Here's how the part is built. I have some questions about the finished solid (model axes, mm). Face numbers are marked on the shaded views. A direction names the side the tool comes from. Round coordinates to 2 decimals unless told otherwise and drop trailing zeros. Write each loop counter-clockwise with the first axis right and the second up, starting at its lowest first coordinate (ties: lowest second). Pieces come first, ordered by that corner, then holes. Notation, with made-up numbers: (6, -20.5) -> (31, -20.5) arc R10 cw to (31, -7.5) -> close; hole circle Ø10 at (-8.5, 73). An arc over 180 degrees is marked (long way). Answer in a Markdown table with one row per item.
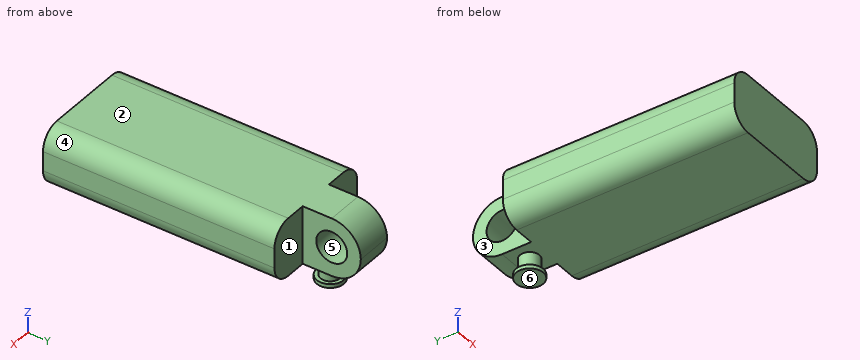
from build123d import *

# Parameters (mm, degrees)
BOSS_EXTRUDE1_DEPTH     = 29.87
SKETCH2_W               = 4.75
SKETCH2_H               = 7.5
BOSS_EXTRUDE2_DEPTH     = 7.5
CUT_EXTRUDE1_DEPTH      = 39.834199168
CUT_EXTRUDE1_DEPTH_BACK = 39.834199168
SKETCH3_R               = 2
SKETCH4_R               = 1.25
BOSS_EXTRUDE3_DEPTH     = 2
SKETCH5_R               = 1.75
BOSS_EXTRUDE4_DEPTH     = 0.5


with BuildPart() as part:
    # Sketch1 → Boss-Extrude1 (new body)
    with BuildSketch(Plane(origin=(0, 0, 0), x_dir=(1, 0, 0), z_dir=(0, 1, 0))):
        with BuildLine():
            Line((-5, 3.75), (5, 3.75))
            ThreePointArc((5, 3.75), (6.767766953, 3.017766953), (7.5, 1.25))
            Line((7.5, 1.25), (7.5, -1.25))
            ThreePointArc((7.5, -1.25), (6.767766953, -3.017766953), (5, -3.75))
            Line((5, -3.75), (-5, -3.75))
            ThreePointArc((-5, -3.75), (-6.767766953, -3.017766953), (-7.5, -1.25))
            Line((-7.5, -1.25), (-7.5, 1.25))
            ThreePointArc((-7.5, 1.25), (-6.767766953, 3.017766953), (-5, 3.75))
        make_face()
    extrude(amount=BOSS_EXTRUDE1_DEPTH)

    # Sketch2 → Boss-Extrude2 (add)
    with BuildSketch(Plane(origin=(0, 29.87, 0), x_dir=(1, 0, 0), z_dir=(0, 1, 0))):
        Rectangle(SKETCH2_W, SKETCH2_H)
    extrude(amount=BOSS_EXTRUDE2_DEPTH)

    # Sketch3 → Cut-Extrude1 (cut, two sides: drawn at the far end of the back side and taken through both)
    with BuildSketch(Plane.ZY.offset(2.375).offset(-CUT_EXTRUDE1_DEPTH_BACK)):
        with BuildLine():
            Line((-3.75, 37.37), (-3.75, 33.62))
            ThreePointArc((-3.75, 33.62), (-2.651650429, 36.271650429), (0, 37.37))
            Line((0, 37.37), (-3.75, 37.37))
        make_face()
        with BuildLine():
            ThreePointArc((0, 37.37), (2.651650429, 36.271650429), (3.75, 33.62))
            Line((3.75, 33.62), (3.75, 37.37))
            Line((3.75, 37.37), (0, 37.37))
        make_face()
        with Locations((0, 33.62)):
            Circle(SKETCH3_R)
    extrude(amount=CUT_EXTRUDE1_DEPTH + CUT_EXTRUDE1_DEPTH_BACK, mode=Mode.SUBTRACT)

    # Sketch4 → Boss-Extrude3 (add)
    with BuildSketch(Plane(origin=(0, 0, -3.75), x_dir=(-1, 0, 0), z_dir=(0, 0, -1))):
        with Locations(Location((0, 31.745, 0), (0, 0, 180))):
            Circle(SKETCH4_R)
    extrude(amount=BOSS_EXTRUDE3_DEPTH)

    # Sketch5 → Boss-Extrude4 (add)
    with BuildSketch(Plane(origin=(0, 0, -5.75), x_dir=(-1, 0, 0), z_dir=(0, 0, -1))):
        with Locations((0, 31.745)):
            Circle(SKETCH5_R)
    extrude(amount=BOSS_EXTRUDE4_DEPTH)


solid = part.part
1) We'd pull the mould along Z, two halves only. Please class the marked faces 4, 5 and 6: +Z half, -Z half, draft (parallel to the pull), parting line (faces both ways), or undercut.
Response:
| item | result |
|---|---|
| face 4 | +Z half |
| face 5 | undercut |
| face 6 | -Z half |
2) I want a section at A-A, the plane x = 0. List the corners of the cut face in (y, z) for me (3 decimals), and give its area (3 significant figures).
Response:
| item | result |
|---|---|
| outline | (0, -3.75) -> (30.495, -3.75) -> (30.495, -5.75) -> (29.995, -5.75) -> (29.995, -6.25) -> (33.495, -6.25) -> (33.495, -5.75) -> (32.995, -5.75) -> (32.995, -3.75) -> (33.62, -3.75) arc R3.75 ccw to (33.62, 3.75) -> (0, 3.75) -> close; hole circle Ø4 at (33.62, 0) |
| area | 268 mm^2 |
3) For pin 1 (2.5 mm diameter, centred on x = 5.5, z = 0.5, fed in from +Y); pin 2 (2 mm diameter, centred on y = 34.5, z = 1, fed in from -X) (3 decimals); pin 3 (5 mm diameter, centred on x = -2, y = 20, fed in from -Z), each with a flat end and sliding along its axis, tell me the tip position at first contact or that it passes through.
Response:
| item | result |
|---|---|
| pin 1 | stops at y = 29.87 |
| pin 2 | stops at x = -2.375 |
| pin 3 | stops at z = -3.75 |
4) Which directions (+Z, -Z, +X, -X, +Y, -Y) give clear straight access to the entire face, cutting with the end or side of a thin tool? Please do the marked faces 1, 2 and 3.
Response:
| item | result |
|---|---|
| face 1 | +Z, -Z, +X, +Y |
| face 2 | +Z, +X, -X, +Y, -Y |
| face 3 | +Z, -Z, -X, +Y |
5) I want a section at D-D, the plane x = 4.5. List the corners of the cut face in (y, z) for me.
Response:
| item | result |
|---|---|
| outline | (0, -3.75) -> (29.87, -3.75) -> (29.87, 3.75) -> (0, 3.75) -> close |
6) I need wall thicknesses on line 1 (Z direction, x = 0.2, y = 33.62); line 2 (Z direction, x = 4, y = 7); line 3 (Y direction, x = -0.5, z = -1). Which ranges of each line are inside material? Lowest first, please. Write a range as [from, to].
Response:
| item | result |
|---|---|
| line 1 | z = [-3.75, -2], [2, 3.75] |
| line 2 | z = [-3.75, 3.75] |
| line 3 | y = [0, 31.89], [35.35, 37.23] |
7) I want a section at B-B, the plane y = 2. List the corners of the cut face in (x, z) for me.
Response:
| item | result |
|---|---|
| outline | (-7.5, -1.25) arc R2.5 ccw to (-5, -3.75) -> (5, -3.75) arc R2.5 ccw to (7.5, -1.25) -> (7.5, 1.25) arc R2.5 ccw to (5, 3.75) -> (-5, 3.75) arc R2.5 ccw to (-7.5, 1.25) -> close |
8) I want a section at C-C, the plane z = -2.5. List the corners of the cut face in (x, y) for me (3 decimals), and give its area (3 significant figures).
Response:
| item | result |
|---|---|
| outline | (-7.165, 0) -> (7.165, 0) -> (7.165, 29.87) -> (2.375, 29.87) -> (2.375, 36.415) -> (-2.375, 36.415) -> (-2.375, 29.87) -> (-7.165, 29.87) -> close |
| area | 459 mm^2 |
